```python
from build123d import *

# Parameters (mm, degrees)
EXTRUDE_1_DEPTH     = 5
SKETCH_2_R          = 3.1
CUT_EXTRUDE_1_DEPTH = 5
SKETCH_3_W          = 46
SKETCH_3_H          = 8
SKETCH_3_W_2        = 80
CUT_EXTRUDE_2_DEPTH = 5
SKETCH_4_R          = 2.1
CUT_EXTRUDE_3_DEPTH = 54.714523176


with BuildPart() as part:
    # 草图1 → 凸台-拉伸1 (new body)
    with BuildSketch(Plane.XY):
        with BuildLine():
            Line((-37, -35.5), (37, -35.5))
            ThreePointArc((37, -35.5), (39.121320344, -34.621320344), (40, -32.5))
            Line((40, -32.5), (40, 32.5))
            ThreePointArc((40, 32.5), (39.121320344, 34.621320344), (37, 35.5))
            Line((37, 35.5), (-37, 35.5))
            ThreePointArc((-37, 35.5), (-39.121320344, 34.621320344), (-40, 32.5))
            Line((-40, 32.5), (-40, -32.5))
            ThreePointArc((-40, -32.5), (-39.121320344, -34.621320344), (-37, -35.5))
        make_face()
    extrude(amount=EXTRUDE_1_DEPTH)

    # 草图2 → 切除-拉伸1 (cut)
    with BuildSketch(Plane.XY.offset(5)):
        with Locations((-31.5, 27)):
            Circle(SKETCH_2_R)
        with Locations((31.5, 27)):
            Circle(SKETCH_2_R)
        with Locations((31.5, -27)):
            Circle(SKETCH_2_R)
        with Locations((-31.5, -27)):
            Circle(SKETCH_2_R)
    extrude(amount=-CUT_EXTRUDE_1_DEPTH, mode=Mode.SUBTRACT)

    # 草图3 → 切除-拉伸2 (cut)
    with BuildSketch(Plane.XY.offset(5)):
        with Locations((0, -35.5)):
            Rectangle(SKETCH_3_W, SKETCH_3_H)
        with Locations((0, 35.5)):
            Rectangle(SKETCH_3_W_2, SKETCH_3_H)
    extrude(amount=-CUT_EXTRUDE_2_DEPTH, mode=Mode.SUBTRACT)

    # 草图4 → 切除-拉伸3 (cut, through all)
    with BuildSketch(Plane.XY.offset(5)):
        with Locations((19, -26)):
            Circle(SKETCH_4_R)
        with Locations((-19, -26)):
            Circle(SKETCH_4_R)
        with Locations((-19, 26)):
            Circle(SKETCH_4_R)
        with Locations((19, 26)):
            Circle(SKETCH_4_R)
    extrude(amount=-CUT_EXTRUDE_3_DEPTH, mode=Mode.SUBTRACT)


solid = part.part
```
The model under review builds one solid part; all positions refer to its coordinate system, in mm. A direction names the side the tool comes from. Round coordinates to 2 decimals unless told otherwise and drop trailing zeros. Write each loop counter-clockwise with the first axis right and the second up, starting at its lowest first coordinate (ties: lowest second). Pieces come first, ordered by that corner, then holes. Notation, with made-up numbers: (-2, 19) - (12, 19) arc R21 ccw to (12, 32) - close; hole circle Ø6 at (5.25, 27). An arc over 180 degrees is marked (long way). Use one line per item in the form item = value.
Q1. Draft analysis for pull direction X (two halves, no side actions). For faces 1 (the flat face through (-40, 0, 2)), 2 (the cylindrical face through (-34.6, -26.9, 2.5)), 3 (the flat face through (-1, 31.5, 3)), state which applies: +X half, -X half, draft (parallel to the pull), parting line (faces both ways), or undercut.
Answer key:
face_1 = -X half
face_2 = undercut
face_3 = draft
Q2. Consider section C-C (y = -26). State the section outline as (x, z) points, and give its area (3 significant figures).
Answer key:
outline = (-40, 0) - (-34.43, 0) - (-34.43, 5) - (-40, 5) - close; (-28.57, 0) - (-21.1, 0) - (-21.1, 5) - (-28.57, 5) - close; (-16.9, 0) - (16.9, 0) - (16.9, 5) - (-16.9, 5) - close; (21.1, 0) - (28.57, 0) - (28.57, 5) - (21.1, 5) - close; (34.43, 0) - (40, 0) - (40, 5) - (34.43, 5) - close
area = 299 mm2
Q3. Insertion check: pin 1 Ø4 at (x, y) = (19, 26) entering from +Z. The pin has a flat end and moves straight along its axis. Give the tip position at first contact, or say it passes through.
Answer key:
pin_1 = through
Q4. Consider section B-B (x = 31.5). State the section outline as (y, z) points.
Answer key:
outline = (-35.5, 0) - (-30.1, 0) - (-30.1, 5) - (-35.5, 5) - close; (-23.9, 0) - (23.9, 0) - (23.9, 5) - (-23.9, 5) - close; (30.1, 0) - (31.5, 0) - (31.5, 5) - (30.1, 5) - close
Q5. Consider section A-A (z = 2.1). State how many separate pieces and enclosed holes the cut face has, and give its area (3 significant figures).
Answer key:
separate_pieces = 1
enclosed_holes = 8
area = 5,000 mm2
Q6. Tool access review of faces 4 (the flat face through (-23, -34, 3)), 5 (the cylindrical face through (29.22, -24.9, 2.54)): name each direction out of +Z, -Z, +X, -X, +Y, -Y from which nothing blocks a thin tool from reaching the whole face with its end or side.
Answer key:
face_4 = +Z, -Z, -Y
face_5 = +Z, -Z
Q7. Consider section D-D (x = 15). State the section outline as (y, z) points, and give its area (3 significant figures).
Answer key:
outline = (-31.5, 0) - (31.5, 0) - (31.5, 5) - (-31.5, 5) - close
area = 315 mm2
Q8. For line 1 (Y direction, x = -31.5, z = 1.8); line 2 (Y direction, x = 33, z = 3.6); line 3 (X direction, y = -25.5, z = 4.25), list the stretches that pass through material, from the lowest coordinate up. Write a range as [from, to].
Answer key:
line_1 = [-35.5, -30.1], [-23.9, 23.9], [30.1, 31.5]
line_2 = [-35.5, -29.71], [-24.29, 24.29], [29.71, 31.5]
line_3 = [-40, -34.21], [-28.79, -21.04], [-16.96, 16.96], [21.04, 28.79], [34.21, 40]
